from build123d import *

# Parameters (mm, degrees)
BOSS_EXTRUDE1_DEPTH = 3


with BuildPart() as part:
    # Sketch3 → Boss-Extrude1 (new body)
    with BuildSketch(Plane(origin=(0, 0, 0), x_dir=(0, 0, -1), z_dir=(1, 0, 0))):
        with BuildLine():
            Line((61.542999323, 28.319708212), (73.742999323, 28.319708212))
            Line((73.742999323, 28.319708212), (73.742999323, 25.319708212))
            Line((73.742999323, 25.319708212), (86.642999323, 25.319708212))
            Line((86.642999323, 25.319708212), (86.642999323, 20.094708212))
            Line((86.642999323, 20.094708212), (84.142999323, 20.094708212))
            ThreePointArc((84.142999323, 20.094708212), (83.289445933, 20.448261603), (83.642999323, 19.594708212))
            Line((83.642999323, 19.594708212), (83.642999323, 8.794708212))
            ThreePointArc((83.642999323, 8.794708212), (83.289445933, 7.941154822), (84.142999323, 8.294708212))
            Line((84.142999323, 8.294708212), (86.642999323, 8.294708212))
            Line((86.642999323, 8.294708212), (86.642999323, 3.069708212))
            Line((86.642999323, 3.069708212), (73.742999323, 3.069708212))
            Line((73.742999323, 3.069708212), (73.742999323, 0.069708212))
            Line((73.742999323, 0.069708212), (61.542999323, 0.069708212))
            Line((61.542999323, 0.069708212), (61.542999323, 3.069708212))
            Line((61.542999323, 3.069708212), (25.242999323, 3.069708212))
            Line((25.242999323, 3.069708212), (25.242999323, 0.069708212))
            Line((25.242999323, 0.069708212), (13.042999323, 0.069708212))
            Line((13.042999323, 0.069708212), (13.042999323, 3.069708212))
            Line((13.042999323, 3.069708212), (0.142999323, 3.069708212))
            Line((0.142999323, 3.069708212), (0.142999323, 8.294708212))
            Line((0.142999323, 8.294708212), (2.642999323, 8.294708212))
            ThreePointArc((2.642999323, 8.294708212), (3.496552714, 7.941154822), (3.142999323, 8.794708212))
            Line((3.142999323, 8.794708212), (3.142999323, 19.594708212))
            ThreePointArc((3.142999323, 19.594708212), (3.496552714, 20.448261603), (2.642999323, 20.094708212))
            Line((2.642999323, 20.094708212), (0.142999323, 20.094708212))
            Line((0.142999323, 20.094708212), (0.142999323, 25.319708212))
            Line((0.142999323, 25.319708212), (13.042999323, 25.319708212))
            Line((13.042999323, 25.319708212), (13.042999323, 28.319708212))
            Line((13.042999323, 28.319708212), (25.242999323, 28.319708212))
            Line((25.242999323, 28.319708212), (25.242999323, 25.319708212))
            Line((25.242999323, 25.319708212), (61.542999323, 25.319708212))
            Line((61.542999323, 25.319708212), (61.542999323, 28.319708212))
        make_face()
    extrude(amount=BOSS_EXTRUDE1_DEPTH)


solid = part.part
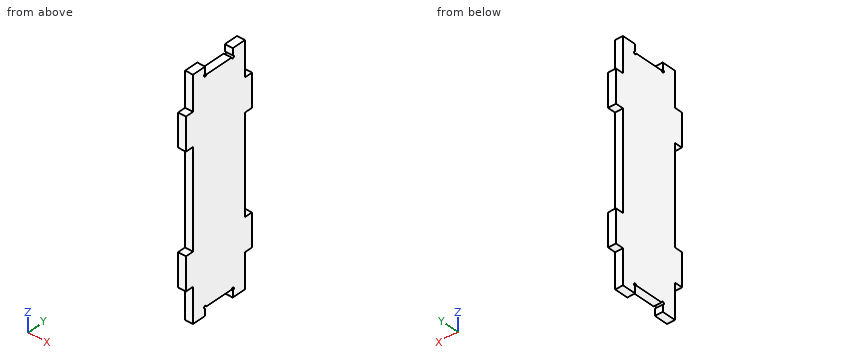
Verification items for the finished model (mm, model axes). Coordinates: 2 decimals unless noted, no trailing zeros. Write each loop counter-clockwise with the first axis right and the second up, starting at its lowest first coordinate (ties: lowest second). Pieces come first, ordered by that corner, then holes. Notation, with made-up numbers: (16, 35) - (35, 35) arc R19 ccw to (35, 60) - close; hole circle Ø10 at (-28.75, 17.25). An arc over 180 degrees is marked (long way). Answer as a JSON object with one key per item and string values.
(1) Cross-section at B-B on y = 15.75. Record the cut outline in (x, z), plus the area to 4 significant figures.
Report:
{"outline": "(0, -83.64) - (3, -83.64) - (3, -3.14) - (0, -3.14) - close", "area": "241.5 mm^2"}
(2) Thickness scan on line 1 along Y through (x, z) = (2.15, -80.5); line 2 along Z through (x, y) = (0.65, 2.75); line 3 along Z through (x, y) = (2.1, 16). Record the ranges inside material, lowest first.
Report:
{"line 1": "3.07 to 25.32", "line 2": "-73.74 to -61.54, -25.24 to -13.04", "line 3": "-83.64 to -3.14"}
(3) Gauge pin test, flat ends, axial feed: pin 1 Ø0.9 at (x, y) = (2, 27.5) entering from -Z; pin 2 Ø0.9 at (x, y) = (2, 13.5) entering from -Z; pin 3 Ø1.5 at (x, y) = (1, 19) entering from +Z. Record the tip position at first contact, or that the pin passes through.
Report:
{"pin 1": "z = -73.74", "pin 2": "z = -83.64", "pin 3": "z = -3.14"}
(4) Cross-section at C-C on z = -9. Record the cut outline in (x, y).
Report:
{"outline": "(0, 3.07) - (3, 3.07) - (3, 25.32) - (0, 25.32) - close"}
